Here's how the part is built. I have some questions about the finished solid (model axes, mm). Face numbers are marked on the shaded views. A direction names the side the tool comes from. Coordinates: 2 decimals unless noted, no trailing zeros. Order: outer loops, then holes, each group sorted by start corner. A loop starts at its lowest first (then second) coordinate and runs counter-clockwise, first axis right, second up. Notation, with made-up numbers: (-2, 0.5) - (14, 0.5) arc R13 ccw to (14, 23.5) - close; hole circle Ø10 at (-14, 60.25). An arc over 180 degrees is marked (long way). Answer in a Markdown table with one row per item. Add a question column.
Item 1: Will these pins go through, and if not, where does the flat tip stop? pin 1 Ø1.4 at (x, z) = (-24, 0) entering from -Y; pin 2 Ø0.8 at (x, z) = (13, 0.5) entering from +Y; pin 3 Ø0.6 at (x, y) = (16.5, 3) entering from +Z.
Item 2: On a 3-axis mill with a long thin cutter (end or side, diameter ignored), from which of +Z, -Z, +X, -X, +Y, -Y can I reach the whole of each face in a straight line? I mean the marked faces 1, 2 and 3. Say none if no direction works.
Item 3: I want a section at B-B (z = 0). Count the separate pieces of the cut face and the enclosed holes in it, plus the area to 3 significant figures.
Item 4: Thinking about a two-plate mould opening in X: for the marked faces 4, 5 and 6, which applies, +X half, -X half, draft (parallel to the pull), parting line (faces both ways), or undercut?
Item 5: I want a section at A-A (y = 1.45). Please give me the cut outline in (x, z), plus the area to 3 significant figures.
Item 6: If I drill on line 1 along Z through (x, y) = (-8.5, 3); line 2 along X through (y, z) = (1.9, 0.7); line 3 along X through (y, z) = (0.4, -1.3), over which ranges is the centre line in solid material (lowest first)? Write a range as from..to.
```python
from build123d import *

# Parameters (mm, degrees)
EXTRUDE_1_DEPTH     = 2.7
EXTRUDE_1_2_DEPTH   = 2.7
EXTRUDE_1_3_DEPTH   = 2.7
EXTRUDE_2_DEPTH     = 0.5
CUT_EXTRUDE_1_REACH = 27.488
SKETCH_2_3_R        = 0.6


with BuildPart() as part:
    # Sketch 1 → Extrude 1 (new body)
    with BuildSketch(Plane(origin=(0, 0, 0), x_dir=(1, 0, 0), z_dir=(0, 1, 0))):
        with BuildLine():
            Line((7.67, -1.5), (13.67, -1.5))
            ThreePointArc((13.67, -1.5), (15.17, 0), (13.67, 1.5))
            Line((13.67, 1.5), (7.67, 1.5))
            ThreePointArc((7.67, 1.5), (6.17, 0), (7.67, -1.5))
        make_face()
    extrude(amount=EXTRUDE_1_DEPTH)



with BuildPart() as body_2:
    # Sketch 1 → Extrude 1 2 (new body)
    with BuildSketch(Plane(origin=(0, 0, 0), x_dir=(1, 0, 0), z_dir=(0, 1, 0))):
        with BuildLine():
            Line((-19.5, 1.5), (-13.5, 1.5))
            ThreePointArc((-13.5, 1.5), (-12, 0), (-13.5, -1.5))
            Line((-13.5, -1.5), (-19.5, -1.5))
            ThreePointArc((-19.5, -1.5), (-21, 0), (-19.5, 1.5))
        make_face()
    extrude(amount=EXTRUDE_1_2_DEPTH)


with BuildPart() as body_3:
    # Sketch 1 → Extrude 1 3 (new body)
    with BuildSketch(Plane(origin=(0, 0, 0), x_dir=(1, 0, 0), z_dir=(0, 1, 0))):
        with BuildLine():
            Line((-3, 1.5), (3, 1.5))
            ThreePointArc((3, 1.5), (4.5, 0), (3, -1.5))
            Line((3, -1.5), (-3, -1.5))
            ThreePointArc((-3, -1.5), (-4.5, 0), (-3, 1.5))
        make_face()
    extrude(amount=EXTRUDE_1_3_DEPTH)


with BuildPart() as part_1:
    add(part.part)

    add(body_2.part)  # Extrude 2 merges body 2

    add(body_3.part)  # Extrude 2 merges body 3
    # Sketch 2 → Extrude 2 (add)
    with BuildSketch(Plane(origin=(0, 2.7, 0), x_dir=(1, 0, 0), z_dir=(0, 1, 0))):
        with BuildLine():
            Line((-24, 1.3), (-22.02, 1.3))
            ThreePointArc((-22.02, 1.3), (-21.843223305, 1.226776695), (-21.77, 1.05))
            Line((-21.77, 1.05), (-21.77, -0.9))
            ThreePointArc((-21.77, -0.9), (-21.682132034, -1.112132034), (-21.47, -1.2))
            Line((-21.47, -1.2), (-20.4, -1.2))
            Line((-20.4, -1.2), (-13.5, 1.5))
            Line((-13.5, 1.5), (-11.52, 1.5))
            ThreePointArc((-11.52, 1.5), (-11.343223305, 1.426776695), (-11.27, 1.25))
            Line((-11.27, 1.25), (-11.27, -0.7))
            ThreePointArc((-11.27, -0.7), (-11.182132034, -0.912132034), (-10.97, -1))
            Line((-10.97, -1), (-9.330662386, -1))
            ThreePointArc((-9.330662386, -1), (-9.722701926, 0.441588043), (-8.5, 1.3))
            Line((-8.5, 1.3), (-5.18, 1.3))
            ThreePointArc((-5.18, 1.3), (-5.003223305, 1.226776695), (-4.93, 1.05))
            Line((-4.93, 1.05), (-4.93, -0.9))
            ThreePointArc((-4.93, -0.9), (-4.842132034, -1.112132034), (-4.63, -1.2))
            Line((-4.63, -1.2), (-3.9, -1.2))
            Line((-3.9, -1.2), (3, 1.5))
            Line((3, 1.5), (5.24, 1.5))
            ThreePointArc((5.24, 1.5), (5.416776695, 1.426776695), (5.49, 1.25))
            Line((5.49, 1.25), (5.49, -0.9))
            ThreePointArc((5.49, -0.9), (5.577867966, -1.112132034), (5.79, -1.2))
            Line((5.79, -1.2), (6.77, -1.2))
            Line((6.77, -1.2), (13.67, 1.5))
            Line((13.67, 1.5), (15.99, 1.5))
            ThreePointArc((15.99, 1.5), (16.166776695, 1.426776695), (16.24, 1.25))
            Line((16.24, 1.25), (16.24, -0.7))
            ThreePointArc((16.24, -0.7), (16.327867966, -0.912132034), (16.54, -1))
            Line((16.54, -1), (17.339337614, -1))
            ThreePointArc((17.339337614, -1), (18.611588043, 1.222701926), (18.17, -1.3))
            Line((18.17, -1.3), (16.19, -1.3))
            ThreePointArc((16.19, -1.3), (16.013223305, -1.226776695), (15.94, -1.05))
            Line((15.94, -1.05), (15.94, 0.9))
            ThreePointArc((15.94, 0.9), (15.852132034, 1.112132034), (15.64, 1.2))
            Line((15.64, 1.2), (14.57, 1.2))
            Line((14.57, 1.2), (7.67, -1.5))
            Line((7.67, -1.5), (5.43, -1.5))
            ThreePointArc((5.43, -1.5), (5.253223305, -1.426776695), (5.18, -1.25))
            Line((5.18, -1.25), (5.18, 0.9))
            ThreePointArc((5.18, 0.9), (5.092132034, 1.112132034), (4.88, 1.2))
            Line((4.88, 1.2), (3.9, 1.2))
            Line((3.9, 1.2), (-3, -1.5))
            Line((-3, -1.5), (-4.98, -1.5))
            ThreePointArc((-4.98, -1.5), (-5.156776695, -1.426776695), (-5.23, -1.25))
            Line((-5.23, -1.25), (-5.23, 0.7))
            ThreePointArc((-5.23, 0.7), (-5.317867966, 0.912132034), (-5.53, 1))
            Line((-5.53, 1), (-7.669337614, 1))
            ThreePointArc((-7.669337614, 1), (-7.277298074, -0.441588043), (-8.5, -1.3))
            Line((-8.5, -1.3), (-11.32, -1.3))
            ThreePointArc((-11.32, -1.3), (-11.496776695, -1.226776695), (-11.57, -1.05))
            Line((-11.57, -1.05), (-11.57, 0.9))
            ThreePointArc((-11.57, 0.9), (-11.657867966, 1.112132034), (-11.87, 1.2))
            Line((-11.87, 1.2), (-12.6, 1.2))
            Line((-12.6, 1.2), (-19.5, -1.5))
            Line((-19.5, -1.5), (-21.82, -1.5))
            ThreePointArc((-21.82, -1.5), (-21.996776695, -1.426776695), (-22.07, -1.25))
            Line((-22.07, -1.25), (-22.07, 0.7))
            ThreePointArc((-22.07, 0.7), (-22.157867966, 0.912132034), (-22.37, 1))
            Line((-22.37, 1), (-23.169337614, 1))
            ThreePointArc((-23.169337614, 1), (-24.441588043, -1.222701926), (-24, 1.3))
        make_face()
    extrude(amount=EXTRUDE_2_DEPTH)

    # Sketch 2_3 → Cut-Extrude 1 (cut, up to next)
    with BuildSketch(Plane(origin=(0, 2.7, 0), x_dir=(1, 0, 0), z_dir=(0, 1, 0)), mode=Mode.PRIVATE) as cut_extrude_1_sk1:
        with Locations(Location((-24, 0, 0), (0, 0, 90))):
            Circle(SKETCH_2_3_R)
    cut_extrude_1_tool1 = extrude(cut_extrude_1_sk1.sketch, amount=CUT_EXTRUDE_1_REACH, mode=Mode.PRIVATE) & part_1.part
    # Sketch 2_3 → Cut-Extrude 1 (cut, up to next)
    with BuildSketch(Plane(origin=(0, 2.7, 0), x_dir=(1, 0, 0), z_dir=(0, 1, 0)), mode=Mode.PRIVATE) as cut_extrude_1_sk2:
        with Locations(Location((-8.5, 0, 0), (0, 0, 90))):
            Circle(SKETCH_2_3_R)
    cut_extrude_1_tool2 = extrude(cut_extrude_1_sk2.sketch, amount=CUT_EXTRUDE_1_REACH, mode=Mode.PRIVATE) & part_1.part
    # Sketch 2_3 → Cut-Extrude 1 (cut, up to next)
    with BuildSketch(Plane(origin=(0, 2.7, 0), x_dir=(1, 0, 0), z_dir=(0, 1, 0)), mode=Mode.PRIVATE) as cut_extrude_1_sk3:
        with Locations(Location((18.17, 0, 0), (0, 0, 90))):
            Circle(SKETCH_2_3_R)
    cut_extrude_1_tool3 = extrude(cut_extrude_1_sk3.sketch, amount=CUT_EXTRUDE_1_REACH, mode=Mode.PRIVATE) & part_1.part
    add(cut_extrude_1_tool1.solids().sort_by_distance((-24, 2.7, 0))[0], mode=Mode.SUBTRACT)
    add(cut_extrude_1_tool2.solids().sort_by_distance((-8.5, 2.7, 0))[0], mode=Mode.SUBTRACT)
    add(cut_extrude_1_tool3.solids().sort_by_distance((18.17, 2.7, 0))[0], mode=Mode.SUBTRACT)


solid = part_1.part
```
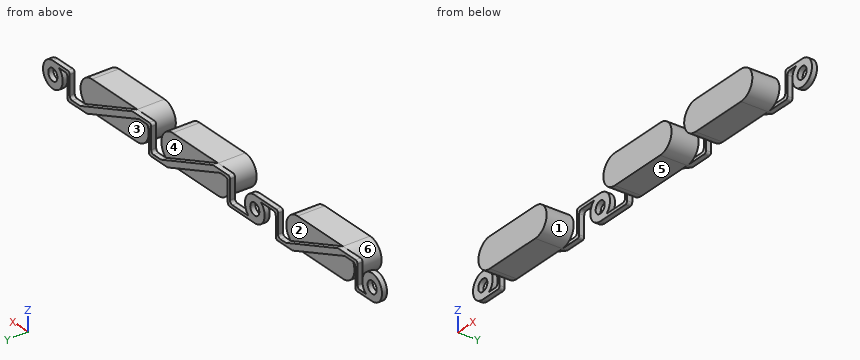
Values follow:
| question | item | result |
|---|---|---|
| 1 | pin 1 | stops at y = 2.7 |
| 1 | pin 2 | stops at y = 2.7 |
| 1 | pin 3 | stops at z = 1.3 |
| 2 | face 1 | -Y |
| 2 | face 2 | +Z, +Y |
| 2 | face 3 | -Z, +Y |
| 3 | separate pieces | 14 |
| 3 | enclosed holes | 0 |
| 3 | area | 78.3 mm^2 |
| 4 | face 4 | undercut |
| 4 | face 5 | draft |
| 4 | face 6 | -X half |
| 5 | outline | (-19.5, -1.5) - (-13.5, -1.5) arc R1.5 ccw to (-13.5, 1.5) - (-19.5, 1.5) arc R1.5 ccw to start; (-3, -1.5) - (3, -1.5) arc R1.5 ccw to (3, 1.5) - (-3, 1.5) arc R1.5 ccw to start; (7.67, -1.5) - (13.67, -1.5) arc R1.5 ccw to (13.67, 1.5) - (7.67, 1.5) arc R1.5 ccw to start |
| 5 | area | 75.2 mm^2 |
| 6 | line 1 | z = -1.3..-0.6, 0.6..1.3 |
| 6 | line 2 | x = -20.83..-12.17, -4.33..4.33, 6.34..15 |
| 6 | line 3 | x = -20.25..-12.75, -3.75..3.75, 6.92..14.42 |
